Could you check a few things on this model? Use its own coordinates, in mm. Face numbers are marked on the shaded views. A direction names the side the tool comes from. Round coordinates to 2 decimals unless told otherwise and drop trailing zeros. Loops run counter-clockwise (first coordinate to the right, second up) from the corner with the lowest first, then second, coordinate; pieces in that order, holes last. Notation, with made-up numbers: (-30.75, -30.5) - (-11.75, -30.5) arc R7 cw to (-11.75, -24.5) - close; hole circle Ø4 at (36, 87). An arc over 180 degrees is marked (long way). Use one line per item in the form item = value.
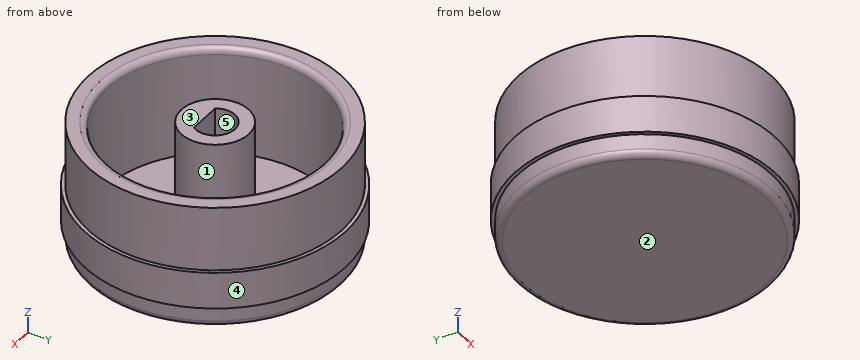
```python
from build123d import *

# Parameters (mm, degrees)
F0_R     = 10.4775
F1_DEPTH = 1.27
F2_R     = 10.4775
F2_R_2   = 8.9535
F2_R_3   = 2.794
F3_DEPTH = 8.89
F4_W     = 0.3048
F4_H     = 3.048
F6_R     = 0.508


with BuildPart() as f1:
    # F0 (on Top) → F1 (new body)
    with BuildSketch(Plane.XY):
        Circle(F0_R)
    extrude(amount=F1_DEPTH)

    # F2 (on face) → F3 (join)
    with BuildSketch(Plane.XY.offset(1.27)):
        Circle(F2_R)
        Circle(F2_R_2, mode=Mode.SUBTRACT)
        Circle(F2_R_3)
        with BuildLine():
            ThreePointArc((-1.397, -0.879882), (0, 1.651), (1.397, -0.879882))
            Line((1.397, -0.879882), (-1.397, -0.879882))
        make_face(mode=Mode.SUBTRACT)
    extrude(amount=F3_DEPTH)

    # F4 (on Right) → F5 (revolve)
    with BuildSketch(Plane.YZ):
        with Locations((10.629893, 3.302)):
            Rectangle(F4_W, F4_H)
    revolve(axis=Axis((0, 0, 0), (0, 0, -1)))

    # F6
    f6_edges = [f1.edges().sort_by_distance(p)[0] for p in [
        (-10.4775, 0, 0),
        (-8.9535, 0, 10.16),
    ]]
    fillet(f6_edges, radius=F6_R)


solid = f1.part
```
1. Please list where these lines run through material, in increasing order: line 1 along Y through (x, z) = (0, 5.5); line 2 along Y through (x, z) = (-1.75, 8.5); line 3 along X through (y, z) = (2, 2).
Solution:
line_1 = -10.48 to -8.95, -2.79 to -0.88, 1.65 to 2.79, 8.95 to 10.48
line_2 = -10.33 to -8.78, -2.18 to 2.18, 8.78 to 10.33
line_3 = -10.6 to -8.73, -1.95 to 1.95, 8.73 to 10.6
2. If we section it at C-C, the plane y = 0: Write out the boundary of the cut face in (x, z).
Solution:
outline = (-10.78, 1.78) - (-10.48, 1.78) - (-10.48, 0.51) arc R0.51 ccw to (-9.97, 0) - (9.97, 0) arc R0.51 ccw to (10.48, 0.51) - (10.48, 1.78) - (10.78, 1.78) - (10.78, 4.83) - (10.48, 4.83) - (10.48, 10.16) - (9.46, 10.16) arc R0.51 ccw to (8.95, 9.65) - (8.95, 1.27) - (2.79, 1.27) - (2.79, 10.16) - (1.65, 10.16) - (1.65, 1.27) - (-1.65, 1.27) - (-1.65, 10.16) - (-2.79, 10.16) - (-2.79, 1.27) - (-8.95, 1.27) - (-8.95, 9.65) arc R0.51 ccw to (-9.46, 10.16) - (-10.48, 10.16) - (-10.48, 4.83) - (-10.78, 4.83) - close
3. If we section it at B-B, the plane x = 0: Write out the boundary of the cut face in (y, z).
Solution:
outline = (-10.78, 1.78) - (-10.48, 1.78) - (-10.48, 0.51) arc R0.51 ccw to (-9.97, 0) - (9.97, 0) arc R0.51 ccw to (10.48, 0.51) - (10.48, 1.78) - (10.78, 1.78) - (10.78, 4.83) - (10.48, 4.83) - (10.48, 10.16) - (9.46, 10.16) arc R0.51 ccw to (8.95, 9.65) - (8.95, 1.27) - (2.79, 1.27) - (2.79, 10.16) - (1.65, 10.16) - (1.65, 1.27) - (-0.88, 1.27) - (-0.88, 10.16) - (-2.79, 10.16) - (-2.79, 1.27) - (-8.95, 1.27) - (-8.95, 9.65) arc R0.51 ccw to (-9.46, 10.16) - (-10.48, 10.16) - (-10.48, 4.83) - (-10.78, 4.83) - close
4. If we section it at A-A, the plane z = 9: Write out the boundary of the cut face in (x, y) (1 decimal).
Solution:
outline = circle Ø21 at (0, 0); circle Ø5.6 at (0, 0); hole circle Ø17.9 at (0, 0); hole (-1.4, -0.9) - (1.4, -0.9) arc R1.7 ccw (long way) to start
5. For P1, Ø1.5, axis at y = -0.5, z = 8.5, coming from the -X side; P2, Ø6, axis at y = -6.5, z = 5.5, coming from the -X side; P3, Ø1.3, axis at x = -0.5, y = 0, coming from the +Z side, each with a flat end and sliding along its axis, tell me the tip position at first contact or that it passes through.
Solution:
P1 = -10.48
P2 = -10.17
P3 = 1.27
6. On a 3-axis mill with a long thin cutter (end or side, diameter ignored), from which of +Z, -Z, +X, -X, +Y, -Y can I reach the whole of each face in a straight line? I mean the marked faces 1 and 2. Say none if no direction works.
Solution:
face_1 = +Z
face_2 = -Z, +X, -X, +Y, -Y
7. We'd pull the mould along Y, two halves only. Please class the marked faces 3, 4 and 5: +Y half, -Y half, draft (parallel to the pull), parting line (faces both ways), or undercut.
Solution:
face_3 = draft
face_4 = parting line
face_5 = undercut
